The model under review builds one solid part; all positions refer to its coordinate system, in mm. A direction names the side the tool comes from. Round coordinates to 2 decimals unless told otherwise and drop trailing zeros. Loops run counter-clockwise (first coordinate to the right, second up) from the corner with the lowest first, then second, coordinate; pieces in that order, holes last. Notation, with made-up numbers: M -25.5,45 L -15.5,45 A12 ccw -15.5,60 Z; hole C 53.5,50 d5. An arc over 180 degrees is marked long. Return JSON: item names as keys, results as strings. Group by question number.
Q1. For faces 1 (the face through (19.1, 1, -1)), 2 (the face through (14, 3, 40.3)), 3 (the face through (0, -2, 40.3)), 4 (the face through (-11.7, 3, -1)), list the 3-axis set-ups (+Z, -Z, +X, -X, +Y, -Y) from which the entire face can be reached by the end or side of a thin tool; tool diameter is ignored.
Q2. Consider section A-A (z = -1). State the section outline as (x, y) points.
Q3. Consider section C-C (x = 15.5). State the section outline as (y, z) points, and give its area (3 significant figures).
Q4. To check wall thickness, follow line 1 along X through (y, z) = (3.25, -35); line 2 along Z through (x, y) = (-12, 2.25); line 3 along Y through (x, z) = (-16.15, -1). State the ranges of each line that lie inside material, in increasing order.
Q5. Consider section D-D (z = -9.5). State the section outline as (x, y) points.
Q6. Clearance check with flat-ended pins moving along their axes: pin 1 Ø5 at (y, z) = (3.5, -2.5) entering from -X; pin 2 Ø5 at (y, z) = (2.5, -0.5) entering from +X; pin 3 Ø2 at (y, z) = (3, -1) entering from -X. State where each tip first meets the part, or that it passes through.
Q7. Consider section B-B (x = 0). State the section outline as (y, z) points, and give its area (3 significant figures).
Q8. Draft analysis for pull direction Z (two halves, no side actions). For faces 5 (the face through (0, -4, 42)), 6 (the face through (-21, 3, 11.65)), 7 (the face through (0, 1, -37.3)), state which applies: pulls with the +Z half, pulls with the -Z half, needs draft (parallel to the pull), parting line crosses it, or undercut.
from build123d import *

# Parameters (mm, degrees)
SALIENTE_EXTRUIR1_DEPTH = 6
CROQUIS2_W              = 10
CROQUIS2_H              = 10
SALIENTE_EXTRUIR2_DEPTH = 3
CORTAR_EXTRUIR1_DEPTH   = 2.4
CORTAR_EXTRUIR2_REACH   = 85.843
CROQUIS4_R              = 1.75
CORTAR_EXTRUIR4_DEPTH   = 2.4
CORTAR_EXTRUIR5_REACH   = 62.207
CROQUIS7_R              = 1.75


with BuildPart() as part:
    # Croquis1 → Saliente-Extruir1 (new body)
    with BuildSketch(Plane(origin=(0, 0, 0), x_dir=(1, 0, 0), z_dir=(0, 1, 0))):
        Polygon((-12.3, 40.3), (-12.3, 37.3), (12.3, 37.3), (12.3, 40.3), (20.3, 40.3), (20.3, 13.65), (19.1, 13.65), (19.1, -11.65), (22.3, -11.65), (22.3, -40.3), (20.3, -40.3), (-20.3, -40.3), (-22.3, -40.3), (-22.3, -11.65), (-19.1, -11.65), (-19.1, 13.65), (-20.3, 13.65), (-20.3, 40.3), align=None)
    extrude(amount=SALIENTE_EXTRUIR1_DEPTH)

    # Croquis2 → Saliente-Extruir2 (add)
    with BuildSketch(Plane.XY.offset(40.3)):
        with Locations((0, 1)):
            Rectangle(CROQUIS2_W, CROQUIS2_H)
    extrude(amount=SALIENTE_EXTRUIR2_DEPTH)

    # Croquis3 → Cortar-Extruir1 (cut)
    with BuildSketch(Plane(origin=(0, 0, -32.3), x_dir=(-1, 0, 0), z_dir=(0, 0, -1))):
        Polygon((1.645448267, 5.85), (3.290896534, 3), (3.290896534, 0), (-3.290896534, 0), (-3.290896534, 3), (-1.645448267, 5.85), (-1.645448267, 6), (1.645448267, 6), align=None)
    extrude(amount=-CORTAR_EXTRUIR1_DEPTH, mode=Mode.SUBTRACT)

    # Croquis4 → Cortar-Extruir2 (cut, up to next)
    with BuildSketch(Plane(origin=(0, 0, -37.3), x_dir=(-1, 0, 0), z_dir=(0, 0, -1)), mode=Mode.PRIVATE) as cortar_extruir2_sk1:
        with Locations((0, 3)):
            Circle(CROQUIS4_R)
    cortar_extruir2_tool1 = extrude(cortar_extruir2_sk1.sketch, amount=-CORTAR_EXTRUIR2_REACH, mode=Mode.PRIVATE) & part.part
    add(cortar_extruir2_tool1.solids().sort_by_distance((0, 3, -37.3))[0], mode=Mode.SUBTRACT)

    # Croquis6 → Cortar-Extruir4 (cut)
    with BuildSketch(Plane.ZY.offset(14.1)):
        Polygon((0.645448267, 5.85), (2.290896534, 3), (2.290896534, 0), (-4.290896534, 0), (-4.290896534, 3), (-2.645448267, 5.85), (-2.645448267, 6), (0.645448267, 6), align=None)
    cortar_extruir4 = extrude(amount=-CORTAR_EXTRUIR4_DEPTH, mode=Mode.SUBTRACT)

    # Croquis7 → Cortar-Extruir5 (cut, up to next)
    with BuildSketch(Plane.ZY.offset(19.1), mode=Mode.PRIVATE) as cortar_extruir5_sk1:
        with Locations((-1, 3)):
            Circle(CROQUIS7_R)
    cortar_extruir5_tool1 = extrude(cortar_extruir5_sk1.sketch, amount=-CORTAR_EXTRUIR5_REACH, mode=Mode.PRIVATE) & part.part
    cortar_extruir5 = cortar_extruir5_tool1.solids().sort_by_distance((-19.1, 3, -1))[0]
    add(cortar_extruir5, mode=Mode.SUBTRACT)

    # Simetría1: Cortar-Extruir4, Cortar-Extruir5 across plane
    add(cortar_extruir4.mirror(Plane(origin=(0, 0, 0), x_dir=(0, 0, 1), z_dir=(1, 0, 0))), mode=Mode.SUBTRACT)
    add(cortar_extruir5.mirror(Plane(origin=(0, 0, 0), x_dir=(0, 0, 1), z_dir=(1, 0, 0))), mode=Mode.SUBTRACT)


solid = part.part
Values:
{
 "1": {"face 1": "+X, +Y, -Y", "face 2": "+Z, +X, +Y, -Y", "face 3": "-Z, +X, -X, -Y", "face 4": "-Y"},
 "2": {"outline": "M -19.1,0 L -14.1,0 L -14.1,1.25 L -19.1,1.25 Z; M -19.1,4.75 L -14.1,4.75 L -14.1,6 L -19.1,6 Z; M -11.7,0 L 11.7,0 L 11.7,6 L -11.7,6 Z; M 14.1,0 L 19.1,0 L 19.1,1.25 L 14.1,1.25 Z; M 14.1,4.75 L 19.1,4.75 L 19.1,6 L 14.1,6 Z"},
 "3": {"outline": "M 0,-40.3 L 6,-40.3 L 6,40.3 L 0,40.3 Z; hole C 3,-1 d3.5", "area": "474 mm2"},
 "4": {"line 1": "x = -20.3 to -1.73, 1.73 to 20.3", "line 2": "z = -37.3 to -4.29, 2.29 to 40.3", "line 3": "y = 0 to 1.25, 4.75 to 6"},
 "5": {"outline": "M -19.1,0 L 19.1,0 L 19.1,6 L -19.1,6 Z"},
 "6": {"pin 1": "stops at x = -19.1", "pin 2": "stops at x = 19.1", "pin 3": "stops at x = -11.7"},
 "7": {"outline": "M -4,40.3 L 0,40.3 L 0,-29.9 L 6,-29.9 L 6,43.3 L -4,43.3 Z; M 0,-37.3 L 1.25,-37.3 L 1.25,-32.3 L 0,-32.3 Z; M 4.75,-37.3 L 6,-37.3 L 6,-32.3 L 4.75,-32.3 Z", "area": "464 mm2"},
 "8": {"face 5": "needs draft", "face 6": "undercut", "face 7": "pulls with the -Z half"}
}
